The model under review builds one solid part; all positions refer to its coordinate system, in mm. A direction names the side the tool comes from. Give positions to 0.01 mm unless a question says otherwise; leave off trailing zeros. Order: outer loops, then holes, each group sorted by start corner. A loop starts at its lowest first (then second) coordinate and runs counter-clockwise, first axis right, second up.
Autodesk Inventor part; units mm, degrees
ref_plane "YZ Plane" through (0, 0, 0) normal (1, 0, 0) x (0, 1, 0)
ref_plane "XZ Plane" through (0, 0, 0) normal (0, 1, 0) x (-1, 0, 0)
ref_plane "XY Plane" through (0, 0, 0) normal (0, 0, 1) x (1, 0, 0)
sketch "Sketch1" plane through (0, 0, 0) normal (0, 0, 1) x (1, 0, 0)
  circle A0 centre (0, 0) radius 6
  dimension "d0" = 12
extrude "Extrusion1" add sketch "Sketch1" along normal blind 2
sketch "Sketch2" plane through (0, 0, 2) normal (0, 0, 1) x (1, 0, 0)
  line L0 (-0.8, -7.5) -> (0.8, -7.5)
  line L1 (0.8, -7.5) -> (0.8, 7.5)
  line L2 (0.8, 7.5) -> (-0.8, 7.5)
  line L3 (-0.8, 7.5) -> (-0.8, -7.5)
  line L4 (-0.8, -7.5) -> (0.8, 7.5) construction
  line L5 (0.8, -7.5) -> (-0.8, 7.5) construction
  circle A0 centre (0, 0) radius 6
  line L6 (-6, 0) -> (6, 0) construction
  point P0 (0.8, 5.9464)
  point P1 (-0.8, 5.9464)
  point P2 (-0.8, -5.9464)
  point P3 (0.8, -5.9464)
  dimension "d5" = 1.6
  dimension "d6" = 15
extrude "Extrusion2" add sketch "Sketch2" along normal blind 1 contours L3 A0 L1
sketch "Sketch3" plane through (0, 0, 0) normal (0, 0, -1) x (-1, 0, 0)
  circle A0 centre (0, 0) radius 3.7
  dimension "d9" = 7.4
extrude "Extrusion3" add sketch "Sketch3" along normal blind 5
sketch "Sketch4" plane through (0, 0, -5) normal (0, 0, -1) x (-1, 0, 0)
  circle A0 centre (0, 0) radius 1.7
  dimension "d12" = 3.4
extrude "Extrusion4" cut sketch "Sketch4" against normal blind 5
properties part number "PrzegubGorny"
1. Insertion check: pin 1 (1.5 mm diameter, centred on x = 1.5, z = 1, fed in from +Y); pin 2 (5.5 mm diameter, centred on x = 2.5, y = 2, fed in from +Z); pin 3 (2.5 mm diameter, centred on x = 0, y = 0, fed in from -Z); pin 4 (1 mm diameter, centred on x = 4, y = -4, fed in from +Z). Each pin has a flat end and moves straight along its axis. Give the tip position at first contact, or say it passes through.
2. Take a section at C-C (z = -3.25). Write out the cut boundary in (x, y).
3. Take a section at D-D (z = 2.25). Write out the cut boundary in (x, y), and give its area (3 significant figures).
4. Take a section at B-B (y = 0). Write out the cut boundary in (x, z), and give its area (3 significant figures).
5. Draft analysis for pull direction X (two halves, no side actions). For faces 1 (the flat face through (3, 0, 2)), 2 (the cylindrical face through (-0.78, -5.95, 1.15)), 3 (the cylindrical face through (0.37, -1.66, -2.54)), 4 (the flat face through (0, 0, 0)), state which applies: pulls with the +X half, pulls with the -X half, needs draft (parallel to the pull), parting line crosses it, or undercut.
6. For faces 5 (the cylindrical face through (0.802, 3.612, -2.465)), 6 (the flat face through (-0.8, 0.1, 2.5)), 7 (the flat face through (0.8, -0.1, 2.5)), list the 3-axis set-ups (+Z, -Z, +X, -X, +Y, -Y) from which the entire face can be reached by the end or side of a thin tool; tool diameter is ignored.
7. Take a section at A-A (x = 0). Write out the cut boundary in (y, z), and give its area (3 significant figures).
8. To check wall thickness, follow line 1 (Y direction, x = 0, z = -2.3); line 2 (Z direction, x = -3, y = 1); line 3 (Z direction, x = -4.25, y = 3.75). State the ranges of each line that lie inside material, in increasing order.
Answer:
1. pin 1: stops at y = 5.95
1. pin 2: stops at z = 3
1. pin 3: stops at z = 0
1. pin 4: stops at z = 2
2. outline: circle Ø7.4 at (0, 0); hole circle Ø3.4 at (0, 0)
3. outline: (-0.8, -5.95) arc R6 ccw to (0.8, -5.95) - (0.8, 5.95) arc R6 ccw to (-0.8, 5.95) - close
3. area: 19.1 mm2
4. outline: (-6, 0) - (-3.7, 0) - (-3.7, -5) - (-1.7, -5) - (-1.7, 0) - (1.7, 0) - (1.7, -5) - (3.7, -5) - (3.7, 0) - (6, 0) - (6, 2) - (0.8, 2) - (0.8, 3) - (-0.8, 3) - (-0.8, 2) - (-6, 2) - close
4. area: 45.6 mm2
5. face 1: needs draft
5. face 2: parting line crosses it
5. face 3: undercut
5. face 4: undercut
6. face 5: -Z
6. face 6: +Z, -X, +Y, -Y
6. face 7: +Z, +X, +Y, -Y
7. outline: (-6, 0) - (-3.7, 0) - (-3.7, -5) - (-1.7, -5) - (-1.7, 0) - (1.7, 0) - (1.7, -5) - (3.7, -5) - (3.7, 0) - (6, 0) - (6, 3) - (-6, 3) - close
7. area: 56.0 mm2
8. line 1: y = -3.7 to -1.7, 1.7 to 3.7
8. line 2: z = -5 to 2
8. line 3: z = 0 to 2
